```python
from build123d import *

# Parameters (mm, degrees)
F1_DEPTH = 38.1
F2_W     = 83.2868572325
F2_H     = 33.5878157057
F2_H_2   = 25.4
F3_DEPTH = 6.35
F4_W     = 46.6631539166
F4_H     = 3.1104013324
F5_DEPTH = 25.4


# Not quite as in the source:
# - a feature names something its author has since deleted; it is built from what else it names


with BuildPart() as f1:
    # F0 (on Front) → F1 (new body)
    with BuildSketch(Plane.XZ):
        Polygon((53.1807057559, 35.5675853789), (-30.1061514765, 35.5675853789), (-30.1061514765, 1.9797696732), (-19.1832855344, 1.9797696732), (-9.4892410561, 1.9797696732), (53.1807057559, 1.9797696732), align=None)
    extrude(amount=-F1_DEPTH)

    # F2 (on face) → F3 (join)
    with BuildSketch(Plane(origin=(0, 38.1, 0), x_dir=(-1, 0, 0), z_dir=(0, 1, 0))):
        with Locations((-11.5372771397, 18.773677526)):
            Rectangle(F2_W, F2_H)
        with Locations((-11.5372771397, -10.7202303268)):
            Rectangle(F2_W, F2_H_2)
    extrude(amount=-F3_DEPTH)

    # F4 (on face) → F5 (cut)
    with BuildSketch(Plane.XY.offset(35.5675853789)):
        with Locations((11.7438416928, 18.4589158744)):
            Rectangle(F4_W, F4_H)
    extrude(amount=-F5_DEPTH, mode=Mode.SUBTRACT)


solid = f1.part
```
Geometry: final body of the model. Coordinates: model frame, mm. A direction names the side the tool comes from. Coordinates: 2 decimals unless noted, no trailing zeros. Order: outer loops, then holes, each group sorted by start corner. A loop starts at its lowest first (then second) coordinate and runs counter-clockwise, first axis right, second up. Notation, with made-up numbers: (48, -14) - (78, -14) arc R28 ccw to (78, 15) - close; hole circle Ø7 at (-25, -7). An arc over 180 degrees is marked (long way). Return JSON: item names as keys, results as strings. Group by question number.
1. Cut plane B-B (x = 25.5). Output: boundary loops of the cut face in (y, z), plus the area to 3 significant figures.
2. Cut plane A-A (z = 31). Output: boundary loops of the cut face in (x, y).
3. Set-up query: faces 5 (the face through (11, 16.904, 23)), 6 (the face through (11, 16, 1.98)), 7 (the face through (12, 35, -23.42)). Return all of +Z, -Z, +X, -X, +Y, -Y with unobstructed straight access to the full face (end or side cutting, diameter ignored); none if empty.
4. Cut plane D-D (y = 26). Output: boundary loops of the cut face in (x, z), plus the area to 3 significant figures.
5. Pull-direction query (Y, two-part tool) for faces 1 (the face through (12, 31.75, -11)), 2 (the face through (53.181, 19, 19)), 3 (the face through (11, 18, 10.168)), 4 (the face through (-11.588, 18, 23)); classes: pulls with the +Y half, pulls with the -Y half, needs draft (parallel to the pull), parting line crosses it, or undercut.
6. Cut plane C-C (z = -3.5). Output: boundary loops of the cut face in (x, y).
7. Material intervals for line 1 along X through (y, z) = (19, 27); line 2 along Y through (x, z) = (28.5, 15); line 3 along Z through (x, y) = (-17, 2.5), sorted ascending. Write a range as [from, to].
Resolved:
{
 "1": {"outline": "(0, 1.98) - (31.75, 1.98) - (31.75, -23.42) - (38.1, -23.42) - (38.1, 35.57) - (20.01, 35.57) - (20.01, 10.17) - (16.9, 10.17) - (16.9, 35.57) - (0, 35.57) - close", "area": "1,360 mm²"},
 "2": {"outline": "(-30.11, 0) - (53.18, 0) - (53.18, 38.1) - (-30.11, 38.1) - close; hole (-11.59, 16.9) - (35.08, 16.9) - (35.08, 20.01) - (-11.59, 20.01) - close"},
 "3": {"face 5": "+Z", "face 6": "-Z, +X, -X, -Y", "face 7": "-Z, +X, -X, +Y, -Y"},
 "4": {"outline": "(-30.11, 1.98) - (53.18, 1.98) - (53.18, 35.57) - (-30.11, 35.57) - close", "area": "2,800 mm²"},
 "5": {"face 1": "pulls with the -Y half", "face 2": "needs draft", "face 3": "undercut", "face 4": "undercut"},
 "6": {"outline": "(-30.11, 31.75) - (53.18, 31.75) - (53.18, 38.1) - (-30.11, 38.1) - close"},
 "7": {"line 1": "x = [-30.11, -11.59], [35.08, 53.18]", "line 2": "y = [0, 16.9], [20.01, 38.1]", "line 3": "z = [1.98, 35.57]"}
}
